For this review, take the finished solid that the model builds, in its own axes (mm). Face numbers are marked on the shaded views. A direction names the side the tool comes from. Give positions to 0.01 mm unless a question says otherwise; leave off trailing zeros. Write each loop counter-clockwise with the first axis right and the second up, starting at its lowest first coordinate (ties: lowest second). Pieces come first, ordered by that corner, then holes. Notation, with made-up numbers: (39, 13.5) -> (76, 13.5) arc R6 ccw to (76, 23.5) -> close; hole circle Ø2 at (-14, 71.25). An arc over 180 degrees is marked (long way). Return JSON: item names as keys, results as strings.
from build123d import *

# Parameters (mm, degrees)
EXTRUDE_1_DEPTH      = 13.5
SKETCH_5_R           = 10.1
CUT_EXTRUDE_2_DEPTH  = 1.5
SKETCH_7_R           = 3.5
CUT_EXTRUDE_3_DEPTH  = 37
SKETCH_21_R          = 4.5
CUT_EXTRUDE_12_DEPTH = 3
SKETCH_9_R           = 1.5
CUT_EXTRUDE_4_DEPTH  = 24.5
SKETCH_11_W          = 60.4
SKETCH_11_H          = 24
EXTRUDE_2_DEPTH      = 10
SKETCH_12_R          = 2.7
CUT_EXTRUDE_5_DEPTH  = 8.5
SKETCH_18_R          = 12
CUT_EXTRUDE_9_DEPTH  = 1.5
SKETCH_19_W          = 16.628747166
SKETCH_19_H          = 6.8
CUT_EXTRUDE_10_DEPTH = 3
SKETCH_20_W          = 76.507524202
SKETCH_20_H          = 37.102074034
CUT_EXTRUDE_11_DEPTH = 3.5


with BuildPart() as part:
    # Sketch 1 → Extrude 1 (new body)
    with BuildSketch(Plane.XY):
        with BuildLine():
            Line((0, 12), (36.185307738, 12))
            Line((36.185307738, 12), (36.185307738, -12))
            Line((36.185307738, -12), (0, -12))
            ThreePointArc((0, -12), (-12, 0), (0, 12))
        make_face()
    extrude(amount=EXTRUDE_1_DEPTH)

    # Sketch 5 → Cut-Extrude 2 (cut)
    with BuildSketch(Plane(origin=(0, 0, 0), x_dir=(-1, 0, 0), z_dir=(0, 0, -1))):
        Circle(SKETCH_5_R)
    extrude(amount=-CUT_EXTRUDE_2_DEPTH, mode=Mode.SUBTRACT)

    # Sketch 7 → Cut-Extrude 3 (cut)
    with BuildSketch(Plane(origin=(0, 0, 1.5), x_dir=(-1, 0, 0), z_dir=(0, 0, -1))):
        Circle(SKETCH_7_R)
    extrude(amount=-CUT_EXTRUDE_3_DEPTH, mode=Mode.SUBTRACT)

    # Sketch 21 → Cut-Extrude 12 (cut)
    with BuildSketch(Plane(origin=(0, 0, 1.5), x_dir=(-1, 0, 0), z_dir=(0, 0, -1))):
        Circle(SKETCH_21_R)
    extrude(amount=-CUT_EXTRUDE_12_DEPTH, mode=Mode.SUBTRACT)

    # Sketch 9 → Cut-Extrude 4 (cut)
    with BuildSketch(Plane(origin=(0, 0, 1.5), x_dir=(-1, 0, 0), z_dir=(0, 0, -1))):
        with Locations((-4.949747468, 4.949747468)):
            Circle(SKETCH_9_R)
        with Locations((4.949747468, 4.949747468)):
            Circle(SKETCH_9_R)
        with Locations((4.949747468, -4.949747468)):
            Circle(SKETCH_9_R)
        with Locations((-4.949747468, -4.949747468)):
            Circle(SKETCH_9_R)
    extrude(amount=-CUT_EXTRUDE_4_DEPTH, mode=Mode.SUBTRACT)


with BuildPart() as body_2:
    # Mirror 14: mirrored copy
    add(part.part.mirror(Plane(origin=(0, 0, -16.7), x_dir=(1, 0, 0), z_dir=(0, 0, -1))))


with BuildPart() as part_1:
    add(part.part)

    add(body_2.part)  # Extrude 2 merges body 2
    # Sketch 11 → Extrude 2 (add)
    with BuildSketch(Plane(origin=(36.185307738, 0, 0), x_dir=(0, 0, -1), z_dir=(1, 0, 0))):
        with Locations((16.7, 0)):
            Rectangle(SKETCH_11_W, SKETCH_11_H)
    extrude(amount=-EXTRUDE_2_DEPTH)

    # Sketch 12 → Cut-Extrude 5 (cut)
    with BuildSketch(Plane.XY.offset(13.5)):
        with Locations((4.949747468, 4.949747468)):
            Circle(SKETCH_12_R)
        with Locations((4.949747468, -4.949747468)):
            Circle(SKETCH_12_R)
        with Locations((-4.949747468, -4.949747468)):
            Circle(SKETCH_12_R)
        with Locations((-4.949747468, 4.949747468)):
            Circle(SKETCH_12_R)
    cut_extrude_5 = extrude(amount=-CUT_EXTRUDE_5_DEPTH, mode=Mode.SUBTRACT)

    # Sketch 18 → Cut-Extrude 9 (cut)
    with BuildSketch(Plane(origin=(0, 0, 0), x_dir=(-1, 0, 0), z_dir=(0, 0, -1))):
        Circle(SKETCH_18_R)
    cut_extrude_9 = extrude(amount=-CUT_EXTRUDE_9_DEPTH, mode=Mode.SUBTRACT)

    # Sketch 19 → Cut-Extrude 10 (cut)
    with BuildSketch(Plane(origin=(0, 0, 1.5), x_dir=(-1, 0, 0), z_dir=(0, 0, -1))):
        with Locations((8.314373583, 0)):
            Rectangle(SKETCH_19_W, SKETCH_19_H)
    cut_extrude_10 = extrude(amount=-CUT_EXTRUDE_10_DEPTH, mode=Mode.SUBTRACT)

    # Sketch 20 → Cut-Extrude 11 (cut)
    with BuildSketch(Plane.XY.offset(13.5)):
        with Locations((20.283666709, 0.248055891)):
            Rectangle(SKETCH_20_W, SKETCH_20_H)
    cut_extrude_11 = extrude(amount=-CUT_EXTRUDE_11_DEPTH, mode=Mode.SUBTRACT)

    # Mirror 24: Cut-Extrude 5, Cut-Extrude 9, Cut-Extrude 10 across plane
    add(cut_extrude_5.mirror(Plane(origin=(0, 0, -16.7), x_dir=(1, 0, 0), z_dir=(0, 0, -1))), mode=Mode.SUBTRACT)
    add(cut_extrude_9.mirror(Plane(origin=(0, 0, -16.7), x_dir=(1, 0, 0), z_dir=(0, 0, -1))), mode=Mode.SUBTRACT)
    add(cut_extrude_10.mirror(Plane(origin=(0, 0, -16.7), x_dir=(1, 0, 0), z_dir=(0, 0, -1))), mode=Mode.SUBTRACT)

    # Mirror 26: Cut-Extrude 11 across plane
    add(cut_extrude_11.mirror(Plane(origin=(0, 0, -16.7), x_dir=(1, 0, 0), z_dir=(0, 0, -1))), mode=Mode.SUBTRACT)


solid = part_1.part
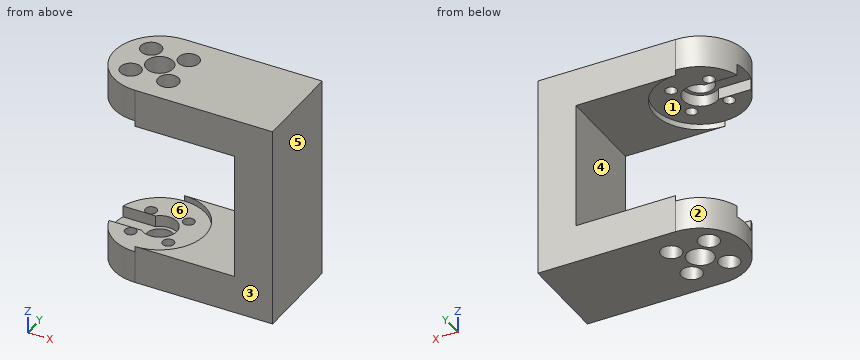
1. Add section A-A, the plane y = 0. State the section outline as (x, z) points.
Results found:
{"outline": "(-12, -43.4) -> (-3.5, -43.4) -> (-3.5, -37.9) -> (-12, -37.9) -> close; (-12, 4.5) -> (-3.5, 4.5) -> (-3.5, 10) -> (-12, 10) -> close; (3.5, -43.4) -> (36.19, -43.4) -> (36.19, 10) -> (3.5, 10) -> (3.5, 4.5) -> (4.5, 4.5) -> (4.5, 1.5) -> (12, 1.5) -> (12, 0) -> (26.19, 0) -> (26.19, -33.4) -> (12, -33.4) -> (12, -34.9) -> (4.5, -34.9) -> (4.5, -37.9) -> (3.5, -37.9) -> close"}
2. The part is to be moulded in two halves that separate along Y. For the marked faces 1, 2 and 3, say which applies: +Y half, -Y half, draft (parallel to the pull), parting line (faces both ways), or undercut.
Results found:
{"face 1": "undercut", "face 2": "parting line", "face 3": "-Y half"}
3. Add section B-B, the plane x = 24. State the section outline as (y, z) points.
Results found:
{"outline": "(-12, -43.4) -> (12, -43.4) -> (12, -33.4) -> (-12, -33.4) -> close; (-12, 0) -> (12, 0) -> (12, 10) -> (-12, 10) -> close"}
4. Add section C-C, the plane z = -40. State the section outline as (x, y) points.
Results found:
{"outline": "(0, -12) -> (36.19, -12) -> (36.19, 12) -> (0, 12) arc R12 ccw to start; hole circle Ø5.4 at (-4.95, -4.95); hole circle Ø5.4 at (-4.95, 4.95); hole circle Ø7 at (0, 0); hole circle Ø5.4 at (4.95, -4.95); hole circle Ø5.4 at (4.95, 4.95)"}
5. For pin 1 (8 mm diameter, centred on x = 0, y = 0, fed in from -Z); pin 2 (8 mm diameter, centred on x = -3.5, z = -30, fed in from +Y); pin 3 (1.6 mm diameter, centred on x = 4.5, y = 4, fed in from -Z); pin 4 (5 mm diameter, centred on x = 4.95, y = -4.95, fed in from +Z), all flat-tipped, find the tip position at first contact; note any pin that passes through.
Results found:
{"pin 1": "stops at z = -43.4", "pin 2": "passes through", "pin 3": "stops at z = -38.4", "pin 4": "stops at z = 5"}
6. Add section D-D, the plane x = -4.5. Count the separate pieces of the cut face and the enclosed holes in it, plus the area to 3 significant figures.
Results found:
{"separate pieces": "6", "enclosed holes": "0", "area": "191 mm²"}
7. To check wall thickness, follow probe 1 along Z at (x, y) = (25, -5.5); probe 2 along Z at (x, y) = (-3.5, 6.5); probe 3 along X at (y, z) = (-5, 3). State the ranges of each line that lie inside material, in increasing order.
Results found:
{"probe 1": "z = -43.4 to -33.4, 0 to 10", "probe 2": "z = -38.4 to -34.9, 1.5 to 5", "probe 3": "x = -10.91 to -6.45, -3.45 to 3.45, 6.45 to 36.19"}
8. For the marked faces 4, 5 and 6, list the 3-axis set-ups (+Z, -Z, +X, -X, +Y, -Y) from which the entire face can be reached by the end or side of a thin tool; tool diameter is ignored.
Results found:
{"face 4": "-X, +Y, -Y", "face 5": "+Z, -Z, +X, +Y, -Y", "face 6": "-X"}
